Work out the finished part from the listing and answer in its coordinate system (mm). A direction names the side the tool comes from. Round coordinates to 2 decimals unless told otherwise and drop trailing zeros. Loops run counter-clockwise (first coordinate to the right, second up) from the corner with the lowest first, then second, coordinate; pieces in that order, holes last.
```python
from build123d import *

# Parameters (mm, degrees)
SKETCH1_W           = 4
SKETCH1_H           = 10
BOSS_EXTRUDE2_DEPTH = 4


with BuildPart() as part:
    # Sketch1 → Boss-Extrude2 (new body)
    with BuildSketch(Plane.XY):
        with BuildLine():
            Line((-30, -27), (-22, -27))
            Line((-22, -27), (-22, -22))
            Line((-22, -22), (-30, -22))
            Line((-30, -22), (-30, 22))
            Line((-30, 22), (-22, 22))
            Line((-22, 22), (-22, 27))
            Line((-22, 27), (-30, 27))
            Line((-30, 27), (-30, 35))
            Line((-30, 35), (-20, 35))
            Line((-20, 35), (-20, 31))
            Line((-20, 31), (-10, 31))
            Line((-10, 31), (-10, 35))
            Line((-10, 35), (10, 35))
            Line((10, 35), (10, 31))
            Line((10, 31), (20, 31))
            Line((20, 31), (20, 35))
            Line((20, 35), (30, 35))
            Line((30, 35), (30, 26.999983113))
            Line((30, 26.999983113), (22, 26.999983113))
            Line((22, 26.999983113), (22, 21.999990545))
            Line((22, 21.999990545), (30, 21.999990545))
            Line((30, 21.999990545), (30, -22))
            Line((30, -22), (22, -22))
            Line((22, -22), (22, -27))
            Line((22, -27), (30, -27))
            Line((30, -27), (30, -31))
            ThreePointArc((30, -31), (28.828427125, -33.828427125), (26, -35))
            Line((26, -35), (-26, -35))
            ThreePointArc((-26, -35), (-28.828427125, -33.828427125), (-30, -31))
            Line((-30, -31), (-30, -27))
        make_face()
        with Locations((-24, 12)):
            Rectangle(SKETCH1_W, SKETCH1_H, mode=Mode.SUBTRACT)
        with Locations((24, 12)):
            Rectangle(SKETCH1_W, SKETCH1_H, mode=Mode.SUBTRACT)
    extrude(amount=BOSS_EXTRUDE2_DEPTH)


solid = part.part
```
1. Given pin 1 (6 mm diameter, centred on x = 17.5, y = 19, fed in from -Z), flat-ended and moving along its own axis, determine where the tip first touches the part or whether it passes through.
Answer key:
pin 1: stops at z = 0
2. Consider probe 1 along Y at (x, z) = (24, 3.45); probe 2 along X at (y, z) = (13, 3); probe 3 along Y at (x, z) = (27, 0.4). Determine where each line is inside the solid, lowest interval first.
Answer key:
probe 1: y = -35 to -27, -22 to 7, 17 to 22, 27 to 35
probe 2: x = -30 to -26, -22 to 22, 26 to 30
probe 3: y = -34.87 to -27, -22 to 22, 27 to 35
3. Which of the six approach directions +Z, -Z, +X, -X, +Y, -Y give full straight-line access (tool end or side, diameter ignored) to faces 4 (the face through (-20, 33, 2)), 5 (the face through (-22, -25, 2)), 6 (the face through (22, 25, 2)), 7 (the face through (-28.797, -33.859, 1.972)), 8 (the face through (-24, 17, 2))?
Answer key:
face 4: +Z, -Z, +Y
face 5: +Z, -Z, -X
face 6: +Z, -Z, +X
face 7: +Z, -Z, -X, -Y
face 8: +Z, -Z
4. Find section A-A (y = 15.5). Write down the section's boundary in (x, z).
Answer key:
outline: (-30, 0) - (-26, 0) - (-26, 4) - (-30, 4) - close; (-22, 0) - (22, 0) - (22, 4) - (-22, 4) - close; (26, 0) - (30, 0) - (30, 4) - (26, 4) - close
5. Find section B-B (x = -23). Write down the section's boundary in (y, z), then the cut area to 3 significant figures.
Answer key:
outline: (-35, 0) - (-27, 0) - (-27, 4) - (-35, 4) - close; (-22, 0) - (7, 0) - (7, 4) - (-22, 4) - close; (17, 0) - (22, 0) - (22, 4) - (17, 4) - close; (27, 0) - (35, 0) - (35, 4) - (27, 4) - close
area: 200 mm2
6. Determine the mould class of faces 1 (the face through (0, 0, 0)), 2 (the face through (-26, -22, 2)), 3 (the face through (28.859, -33.797, 1.972)) for opening direction Y: +Y half, -Y half, draft (parallel to the pull), parting line (faces both ways), or undercut.
Answer key:
face 1: draft
face 2: undercut
face 3: -Y half
7. Find section C-C (z = 1.5). Give the number of separate pieces and of enclosed holes in the cut face, then the cut area to 3 significant figures.
Answer key:
separate pieces: 1
enclosed holes: 2
area: 3,870 mm2
8. Find section D-D (x = -11). Write down the section's boundary in (y, z).
Answer key:
outline: (-35, 0) - (31, 0) - (31, 4) - (-35, 4) - close
